from build123d import *

# Parameters (mm, degrees)
BOSS_EXTRUDE1_DEPTH = 30
BOSS_EXTRUDE2_DEPTH = 10.2
CUT_EXTRUDE1_DEPTH  = 10.2


with BuildPart() as part:
    # Sketch1 → Boss-Extrude1 (new body)
    with BuildSketch(Plane(origin=(0, 0, 0), x_dir=(1, 0, 0), z_dir=(0, 1, 0))):
        Polygon((18.1, 3.1), (18.1, 5.1), (22.1, 5.1), (22.1, -5.1), (-22.1, -5.1), (-22.1, 5.1), (-18.1, 5.1), (-20.1, 3.1), (-20.1, -3.1), (20.1, -3.1), (20.1, 3.1), align=None)
    extrude(amount=BOSS_EXTRUDE1_DEPTH)

    # Sketch2 → Boss-Extrude2 (add)
    with BuildSketch(Plane.XY.offset(5.1)):
        Polygon((47.02820323, 34), (29.02820323, 65.176914536), (22.1, 61.176914536), (22.1, 30), (22.1, 0), (40.1, 30), align=None)
    extrude(amount=-BOSS_EXTRUDE2_DEPTH)

    # Sketch3 → Cut-Extrude1 (cut)
    with BuildSketch(Plane.XY.offset(5.1)):
        Polygon((44.346152423, 34.645448267), (28.246152423, 62.531466269), (27.033716857, 61.831466269), (28.833716857, 58.713774815), (25.369615242, 56.713774815), (37.869615242, 35.063139721), (41.333716857, 37.063139721), (43.133716857, 33.945448267), align=None)
    extrude(amount=-CUT_EXTRUDE1_DEPTH, mode=Mode.SUBTRACT)


solid = part.part
Verification items for the finished model (mm, model axes). A direction names the side the tool comes from. Give positions to 0.01 mm unless a question says otherwise; leave off trailing zeros. Order: outer loops, then holes, each group sorted by start corner. A loop starts at its lowest first (then second) coordinate and runs counter-clockwise, first axis right, second up. Notation, with made-up numbers: (78.5, -24) -> (91.5, -24) arc R24 cw to (91.5, -9) -> close; hole circle Ø10 at (19, -22.5). An arc over 180 degrees is marked (long way). Answer as CSV lines item,"result".
Q1. Access from +Z, -Z, +X, -X, +Y, -Y to the whole of each face (thin tool, end or side, straight path). Record for faces 1 (the flat face through (0.1, 0, 3.4)), 2 (the flat face through (42.22, 35.53, 0.07)), 3 (the flat face through (22.1, 46, 0)), 4 (the flat face through (18.1, 15, -4)), 5 (the flat face through (-20.1, 15, 0)).
Solutions:
face 1,"+Z, -Z, +X, -X, -Y"
face 2,"+Z, -Z"
face 3,"+Z, -Z, -X, +Y"
face 4,"-Z, +Y, -Y"
face 5,"+Y, -Y"
Q2. Sectioned sample at C-C on y = 41. Record the cut outline in (x, z), plus the area to 3 significant figures.
Solutions:
outline,"(22.1, -5.1) -> (34.44, -5.1) -> (34.44, 5.1) -> (22.1, 5.1) -> close; (40.68, -5.1) -> (42.99, -5.1) -> (42.99, 5.1) -> (40.68, 5.1) -> close"
area,"149 mm²"
Q3. Sectioned sample at D-D on x = 21. Record the cut outline in (y, z).
Solutions:
outline,"(0, -5.1) -> (30, -5.1) -> (30, 5.1) -> (0, 5.1) -> close"
Q4. Sectioned sample at A-A on z = -0.5. Record the cut outline in (x, y), plus the area to 3 significant figures.
Solutions:
outline,"(-22.1, 0) -> (-20.1, 0) -> (-20.1, 30) -> (-22.1, 30) -> close; (20.1, 0) -> (22.1, 0) -> (40.1, 30) -> (47.03, 34) -> (29.03, 65.18) -> (22.1, 61.18) -> (22.1, 30) -> (20.1, 30) -> close; hole (25.37, 56.71) -> (37.87, 35.06) -> (41.33, 37.06) -> (43.13, 33.95) -> (44.35, 34.65) -> (28.25, 62.53) -> (27.03, 61.83) -> (28.83, 58.71) -> close"
area,"814 mm²"
Q5. Sectioned sample at B-B on y = 12. Record the cut outline in (x, z).
Solutions:
outline,"(-22.1, -5.1) -> (-18.1, -5.1) -> (-20.1, -3.1) -> (-20.1, 3.1) -> (20.1, 3.1) -> (20.1, -3.1) -> (18.1, -3.1) -> (18.1, -5.1) -> (29.3, -5.1) -> (29.3, 5.1) -> (-22.1, 5.1) -> close"
Q6. Depth check by flat-ended pin: pin 1 (15 mm diameter, centred on x = -6.5, y = 20, fed in from -Z); pin 2 (5 mm diameter, centred on x = 11, y = 33.5, fed in from +Z); pin 3 (5 mm diameter, centred on y = 41.5, z = -2, fed in from +X); pin 4 (1.9 mm diameter, centred on y = 18, z = -1.5, fed in from +X). Enter the tip coordinate at first touch or a pass-through.
Solutions:
pin 1,"stops at z = 3.1"
pin 2,"passes through"
pin 3,"stops at x = 44.14"
pin 4,"stops at x = 33.47"
Q7. Scan lines: probe 1 along Z at (x, y) = (-12, 21.5); probe 2 along Y at (x, z) = (38, -2.75); probe 3 along Y at (x, z) = (11.5, 4.5). Record each from-to range of solid material in increasing order.
Solutions:
probe 1,"z = 3.1 to 5.1"
probe 2,"y = 26.5 to 35.14, 45.64 to 49.64"
probe 3,"y = 0 to 30"
Q8. Release check for a two-part mould opening along X. For faces 6 (the flat face through (27.13, 57.73, 0.07)), 7 (the flat face through (43.516, 31.972, 0.071)), 8 (the flat face through (0.1, 30, 3.4)) record: +X half, -X half, draft (parallel to the pull), parting line (faces both ways), or undercut.
Solutions:
face 6,"undercut"
face 7,"+X half"
face 8,"draft"
